For this review, take the finished solid that the model builds, in its own axes (mm). Face numbers are marked on the shaded views. A direction names the side the tool comes from. Give positions to 0.01 mm unless a question says otherwise; leave off trailing zeros. Loops run counter-clockwise (first coordinate to the right, second up) from the corner with the lowest first, then second, coordinate; pieces in that order, holes last. Notation, with made-up numbers: (43, 59.25) - (58, 59.25) arc R30 ccw to (58, 93.25) - close; hole circle Ø2 at (-12.5, 0). An arc over 180 degrees is marked (long way). Answer in a Markdown table with one row per item.
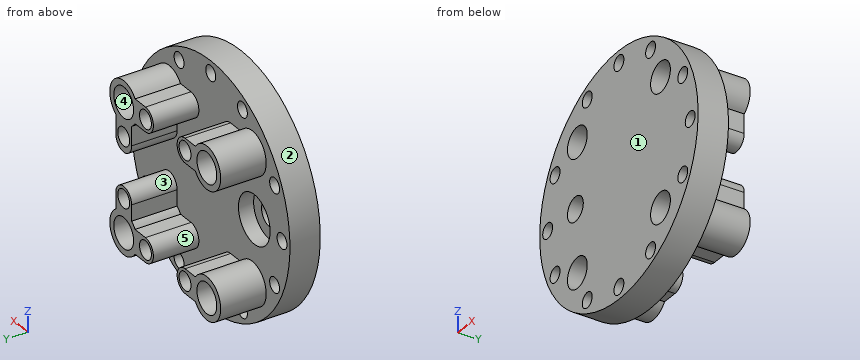
```python
from build123d import *

# Parameters (mm, degrees)
SKETCH1_R           = 40
SKETCH1_R_2         = 5
SKETCH1_R_3         = 5.000393793
SKETCH1_R_4         = 2.5
SKETCH1_R_5         = 2.500004974
SKETCH1_R_6         = 2.503537869
BOSS_EXTRUDE4_DEPTH = 10
SKETCH2_R           = 4
CUT_EXTRUDE1_DEPTH  = 10
SKETCH3_R           = 8
CUT_EXTRUDE2_DEPTH  = 5
SKETCH4_R           = 3
SKETCH4_R_2         = 7
SKETCH4_R_3         = 5
SKETCH4_R_4         = 5.000393793
BOSS_EXTRUDE9_DEPTH = 15


with BuildPart() as part:
    # Sketch1 → Boss-Extrude4 (new body)
    with BuildSketch(Plane(origin=(0, 0, 0), x_dir=(1, 0, 0), z_dir=(0, 1, 0))):
        with Locations(Location((0, 0, 0), (0, 0, 270))):
            Circle(SKETCH1_R)
        with Locations(Location((-21, 21, 0), (0, 0, 270))):
            Circle(SKETCH1_R_2, mode=Mode.SUBTRACT)
        with Locations(Location((-21, -21, 0), (0, 0, 270))):
            Circle(SKETCH1_R_3, mode=Mode.SUBTRACT)
        with Locations(Location((21, -21, 0), (0, 0, 270))):
            Circle(SKETCH1_R_2, mode=Mode.SUBTRACT)
        with Locations(Location((21, 21, 0), (0, 0, 270))):
            Circle(SKETCH1_R_2, mode=Mode.SUBTRACT)
        with Locations(Location((36, 0, 0), (0, 0, 270))):
            Circle(SKETCH1_R_4, mode=Mode.SUBTRACT)
        with Locations(Location((0, 36, 0), (0, 0, 270))):
            Circle(SKETCH1_R_4, mode=Mode.SUBTRACT)
        with Locations(Location((0, -36, 0), (0, 0, 270))):
            Circle(SKETCH1_R_4, mode=Mode.SUBTRACT)
        with Locations(Location((16, 32.25, 0), (0, 0, 270))):
            Circle(SKETCH1_R_4, mode=Mode.SUBTRACT)
        with Locations(Location((-16, 32.25, 0), (0, 0, 270))):
            Circle(SKETCH1_R_4, mode=Mode.SUBTRACT)
        with Locations(Location((-32.25, 16, 0), (0, 0, 270))):
            Circle(SKETCH1_R_4, mode=Mode.SUBTRACT)
        with Locations(Location((-32.25, -16.004986802, 0), (0, 0, 270))):
            Circle(SKETCH1_R_5, mode=Mode.SUBTRACT)
        with Locations(Location((-16, -32.25, 0), (0, 0, 270))):
            Circle(SKETCH1_R_4, mode=Mode.SUBTRACT)
        with Locations(Location((16, -32.25, 0), (0, 0, 270))):
            Circle(SKETCH1_R_4, mode=Mode.SUBTRACT)
        with Locations(Location((32.25, 16, 0), (0, 0, 270))):
            Circle(SKETCH1_R_4, mode=Mode.SUBTRACT)
        with Locations(Location((32.25, -16.004986802, 0), (0, 0, 270))):
            Circle(SKETCH1_R_6, mode=Mode.SUBTRACT)
        with Locations(Location((-36, 0, 0), (0, 0, 270))):
            Circle(SKETCH1_R_4, mode=Mode.SUBTRACT)
    extrude(amount=BOSS_EXTRUDE4_DEPTH)

    # Sketch2 → Cut-Extrude1 (cut)
    with BuildSketch(Plane(origin=(0, 10, 0), x_dir=(1, 0, 0), z_dir=(0, 1, 0))):
        with Locations(Location((-22, 0, 0), (0, 0, 270))):
            Circle(SKETCH2_R)
    extrude(amount=-CUT_EXTRUDE1_DEPTH, mode=Mode.SUBTRACT)

    # Sketch3 → Cut-Extrude2 (cut)
    with BuildSketch(Plane(origin=(0, 10, 0), x_dir=(1, 0, 0), z_dir=(0, 1, 0))):
        with Locations(Location((-22, 0, 0), (0, 0, 270))):
            Circle(SKETCH3_R)
    extrude(amount=-CUT_EXTRUDE2_DEPTH, mode=Mode.SUBTRACT)

    # Sketch4 → Boss-Extrude9 (add)
    # profile 1 of 10: a face of its own
    with BuildSketch(Plane(origin=(0, 10, 0), x_dir=(1, 0, 0), z_dir=(0, 1, 0))):
        with BuildLine():
            Line((-15.255437353, 17), (-10, 17))
            ThreePointArc((-10, 17), (-6, 21), (-10, 25))
            Line((-10, 25), (-15.255437353, 25))
            ThreePointArc((-15.255437353, 25), (-14.321229959, 23.096194346), (-14, 21))
            ThreePointArc((-14, 21), (-14.321229959, 18.903805654), (-15.255437353, 17))
        make_face()
        with Locations(Location((-10, 21, 0), (0, 0, 270))):
            Circle(SKETCH4_R, mode=Mode.SUBTRACT)
    # profile 2 of 10: a face of its own
    with BuildSketch(Plane(origin=(0, 10, 0), x_dir=(1, 0, 0), z_dir=(0, 1, 0))):
        with Locations((-21, 21)):
            Circle(SKETCH4_R_2)
        with Locations(Location((-21, 21, 0), (0, 0, 270))):
            Circle(SKETCH4_R_3, mode=Mode.SUBTRACT)
    # profile 3 of 10: a face of its own
    with BuildSketch(Plane(origin=(0, 10, 0), x_dir=(1, 0, 0), z_dir=(0, 1, 0))):
        with Locations((-21, -21)):
            Circle(SKETCH4_R_2)
        with Locations(Location((-21, -21, 0), (0, 0, 270))):
            Circle(SKETCH4_R_4, mode=Mode.SUBTRACT)
    # profile 4 of 10: a face of its own
    with BuildSketch(Plane(origin=(0, 10, 0), x_dir=(1, 0, 0), z_dir=(0, 1, 0))):
        with BuildLine():
            ThreePointArc((-10, -25), (-6, -21), (-10, -17))
            Line((-10, -17), (-15.255437353, -17))
            ThreePointArc((-15.255437353, -17), (-14.321229959, -18.903805654), (-14, -21))
            ThreePointArc((-14, -21), (-14.321229959, -23.096194346), (-15.255437353, -25))
            Line((-15.255437353, -25), (-10, -25))
        make_face()
        with Locations(Location((-10, -21, 0), (0, 0, 270))):
            Circle(SKETCH4_R, mode=Mode.SUBTRACT)
    # profile 5 of 10: a face of its own
    with BuildSketch(Plane(origin=(0, 10, 0), x_dir=(1, 0, 0), z_dir=(0, 1, 0))):
        with Locations((21, -21)):
            Circle(SKETCH4_R_2)
        with Locations(Location((21, -21, 0), (0, 0, 270))):
            Circle(SKETCH4_R_3, mode=Mode.SUBTRACT)
    # profile 6 of 10: a face of its own
    with BuildSketch(Plane(origin=(0, 10, 0), x_dir=(1, 0, 0), z_dir=(0, 1, 0))):
        with BuildLine():
            ThreePointArc((10, -17), (6, -21), (10, -25))
            Line((10, -25), (15.255437353, -25))
            ThreePointArc((15.255437353, -25), (14, -21), (15.255437353, -17))
            Line((15.255437353, -17), (10, -17))
        make_face()
        with Locations(Location((10, -21, 0), (0, 0, 270))):
            Circle(SKETCH4_R, mode=Mode.SUBTRACT)
    # profile 7 of 10: a face of its own
    with BuildSketch(Plane(origin=(0, 10, 0), x_dir=(1, 0, 0), z_dir=(0, 1, 0))):
        with BuildLine():
            Line((17, -9), (17, -15.255437353))
            ThreePointArc((17, -15.255437353), (21, -14), (25, -15.255437353))
            Line((25, -15.255437353), (25, -9))
            ThreePointArc((25, -9), (21, -5), (17, -9))
        make_face()
        with Locations(Location((21, -10, 0), (0, 0, 270))):
            Circle(SKETCH4_R, mode=Mode.SUBTRACT)
    # profile 8 of 10: a face of its own
    with BuildSketch(Plane(origin=(0, 10, 0), x_dir=(1, 0, 0), z_dir=(0, 1, 0))):
        with Locations((21, 21)):
            Circle(SKETCH4_R_2)
        with Locations(Location((21, 21, 0), (0, 0, 270))):
            Circle(SKETCH4_R_3, mode=Mode.SUBTRACT)
    # profile 9 of 10: a face of its own
    with BuildSketch(Plane(origin=(0, 10, 0), x_dir=(1, 0, 0), z_dir=(0, 1, 0))):
        with BuildLine():
            Line((25, 10), (25, 15.255437353))
            ThreePointArc((25, 15.255437353), (21, 14), (17, 15.255437353))
            Line((17, 15.255437353), (17, 10))
            ThreePointArc((17, 10), (21, 6), (25, 10))
        make_face()
        with Locations(Location((21, 10, 0), (0, 0, 270))):
            Circle(SKETCH4_R, mode=Mode.SUBTRACT)
    # profile 10 of 10: a face of its own
    with BuildSketch(Plane(origin=(0, 10, 0), x_dir=(1, 0, 0), z_dir=(0, 1, 0))):
        with BuildLine():
            Line((15.255437353, 25), (10, 25))
            ThreePointArc((10, 25), (6, 21), (10, 17))
            Line((10, 17), (15.255437353, 17))
            ThreePointArc((15.255437353, 17), (14, 21), (15.255437353, 25))
        make_face()
        with Locations(Location((10, 21, 0), (0, 0, 270))):
            Circle(SKETCH4_R, mode=Mode.SUBTRACT)
    extrude(amount=BOSS_EXTRUDE9_DEPTH)


solid = part.part
```
1. Mouldability with a two-part tool opening along Z and no side actions: class the marked faces 1, 2 and 3 as released by +Z, released by -Z, zero draft, split by the parting line, or undercut.
Values:
| item | result |
|---|---|
| face 1 | zero draft |
| face 2 | split by the parting line |
| face 3 | undercut |
2. Wall thickness on line 1 (X direction, y = 5.25, z = 0); line 2 (X direction, y = 21, z = 21); line 3 (X direction, y = 8, z = -32.25): over which ranges is each line inside the solid? List them lowest first. Write a range as [from, to].
Values:
| item | result |
|---|---|
| line 1 | x = [-40, -38.5], [-33.5, -30], [-14, 33.5], [38.5, 40] |
| line 2 | x = [-28, -26], [-16, -13], [-7, -6], [6, 7], [13, 16], [26, 28] |
| line 3 | x = [-23.66, -18.5], [-13.5, 13.5], [18.5, 23.66] |
3. Clearance check with flat-ended pins moving along their axes: pin 1 (3 mm diameter, centred on y = 20.5, z = 13.5, fed in from -X); pin 2 (2 mm diameter, centred on y = 18.5, z = -6.5, fed in from -X); pin 3 (1 mm diameter, centred on y = 17, z = -25, fed in from +X); pin 4 (1 mm diameter, centred on x = -15.5, z = -30.5, fed in from +Y). State where each tip first meets the part, or that it passes through.
Values:
| item | result |
|---|---|
| pin 1 | stops at x = -24.61 |
| pin 2 | stops at x = 17.88 |
| pin 3 | stops at x = 27.06 |
| pin 4 | passes through |
4. For the marked faces 4 and 5, list the 3-axis set-ups (+Z, -Z, +X, -X, +Y, -Y) from which the entire face can be reached by the end or side of a thin tool; tool diameter is ignored.
Values:
| item | result |
|---|---|
| face 4 | +Y, -Y |
| face 5 | +Y |
5. We need section A-A, the plane y = 20. Count the separate pieces of the cut face and the enclosed holes in it, and give its area (3 significant figures).
Values:
| item | result |
|---|---|
| separate pieces | 4 |
| enclosed holes | 10 |
| area | 502 mm^2 |
6. We need section D-D, the plane z = 36. Give the boundary of the cut face in (x, y).
Values:
| item | result |
|---|---|
| outline | (-17.44, 0) - (-2.5, 0) - (-2.5, 10) - (-17.44, 10) - close; (2.5, 0) - (17.44, 0) - (17.44, 10) - (2.5, 10) - close |
7. We need section B-B, the plane z = -32.25. Give the boundary of the cut face in (x, y).
Values:
| item | result |
|---|---|
| outline | (-23.66, 0) - (-18.5, 0) - (-18.5, 10) - (-23.66, 10) - close; (-13.5, 0) - (13.5, 0) - (13.5, 10) - (-13.5, 10) - close; (18.5, 0) - (23.66, 0) - (23.66, 10) - (18.5, 10) - close |
8. We need section C-C, the plane x = -22. Give the boundary of the cut face in (y, z).
Values:
| item | result |
|---|---|
| outline | (0, -33.41) - (10, -33.41) - (10, -27.93) - (25, -27.93) - (25, -25.9) - (0, -25.9) - close; (0, -16.1) - (25, -16.1) - (25, -14.07) - (10, -14.07) - (10, -8) - (5, -8) - (5, -4) - (0, -4) - close; (0, 4) - (5, 4) - (5, 8) - (10, 8) - (10, 14.07) - (25, 14.07) - (25, 16.1) - (0, 16.1) - close; (0, 25.9) - (25, 25.9) - (25, 27.93) - (10, 27.93) - (10, 33.41) - (0, 33.41) - close |
